```python
from build123d import *

# Parameters (mm, degrees)
F0_W        = 25
F0_H        = 25
F1_DEPTH    = 6
F2_W        = 13
F2_H        = 3
F3_DEPTH    = 25
F4_T1_DEPTH = 50.7168298797
F4_T3_DEPTH = 50.7168298797


# Not quite as in the source:
# - a fillet or chamfer that OpenCascade refuses, or shapes differently, is made with other operations: its cross-section is extruded or revolved along the edge and cut away or added


with BuildPart() as f1:
    # F0 (on Top) → F1 (new body)
    with BuildSketch(Plane.XY):
        with Locations((-12.5, 12.5)):
            Rectangle(F0_W, F0_H)
    extrude(amount=F1_DEPTH)

    # F2 (on face) → F3 (cut)
    with BuildSketch(Plane(origin=(-25, 0, 0), x_dir=(0, -1, 0), z_dir=(-1, 0, 0))):
        with Locations((-12.5, 3)):
            Rectangle(F2_W, F2_H)
    extrude(amount=-F3_DEPTH, mode=Mode.SUBTRACT)

    # F4: chamfer of 5 on 4 edges, made by hand

    # F4_s2 → F4_t1 (cut)
    with BuildSketch(Plane.YZ.offset(-37.8584149398)):
        Polygon((0, 1), (5, 6), (0, 6), align=None)
        Polygon((20, 6), (25, 1), (25, 6), align=None)
    extrude(amount=F4_T1_DEPTH, mode=Mode.SUBTRACT)

    # F4_s4 → F4_t3 (cut)
    with BuildSketch(Plane.XZ.offset(-37.8584149398)):
        Polygon((-25, 1), (-20, 6), (-25, 6), align=None)
        Polygon((0, 1), (-5, 6), (0, 6), align=None)
    extrude(amount=F4_T3_DEPTH, mode=Mode.SUBTRACT)


solid = f1.part
```
CAD build for the part. Positions are in the model's coordinates, mm. A direction names the side the tool comes from. Round coordinates to 2 decimals unless told otherwise and drop trailing zeros. Loops run counter-clockwise (first coordinate to the right, second up) from the corner with the lowest first, then second, coordinate; pieces in that order, holes last. Notation, with made-up numbers: M 76.5,64.25 L 100.5,64.25 A12 cw 100.5,77.25 Z; hole C 70,84 d7. An arc over 180 degrees is marked long. Return JSON: item names as keys, results as strings. Group by question number.
(1) Saw through at C-C, the plane x = -22.25. List the corners of the cut face in (y, z).
(2) Saw through at B-B, the plane z = 3.75. List the corners of the cut face in (x, y), and give its area (3 significant figures).
(3) Mould opens along Y. For faces 1 (the flat face through (-13, 13, 1.5)), 2 (the flat face through (-4, 13, 5)), 3 (the flat face through (-13, 22, 4)), 4 (the flat face through (-13, 2, 3)) say: +Y half, -Y half, draft (parallel to the pull), parting line (faces both ways), or undercut.
(4) Saw through at D-D, the plane x = -11.5. List the corners of the cut face in (y, z).
(5) Saw through at A-A, the plane y = 12.25. List the corners of the cut face in (x, z), and give its area (3 significant figures).
(6) Wall check: probe 1 along Z at (x, y) = (-15.5, 7.5); probe 2 along Z at (x, y) = (-22.75, 15); probe 3 along Z at (x, y) = (-18.75, 21.5). Give the ranges that are in metal, low to high. Write a range as [from, to].
(7) Tool access for faces 5 (the flat face through (-13, 19, 3)), 6 (the flat face through (-13, 13, 0)): list every direction of +Z, -Z, +X, -X, +Y, -Y with a clear straight run to the whole face (end or side of a thin tool).
(8) Drop flat-ended pins along their axis: P1, Ø2.5, axis at x = -6.5, z = 2.5, coming from the -Y side; P2, Ø1.5, axis at x = -22.5, z = 3, coming from the -Y side. Give the stop position or say it passes through.
Answer list:
{
 "1": {"outline": "M 0,0 L 25,0 L 25,1 L 22.25,3.75 L 19,3.75 L 19,1.5 L 6,1.5 L 6,3.75 L 2.75,3.75 L 0,1 Z"},
 "2": {"outline": "M -22.25,2.75 L -2.75,2.75 L -2.75,6 L -22.25,6 Z; M -22.25,19 L -2.75,19 L -2.75,22.25 L -22.25,22.25 Z", "area": "127 mm2"},
 "3": {"face 1": "undercut", "face 2": "draft", "face 3": "+Y half", "face 4": "-Y half"},
 "4": {"outline": "M 0,0 L 25,0 L 25,1 L 20,6 L 5,6 L 0,1 Z; hole M 6,1.5 L 19,1.5 L 19,4.5 L 6,4.5 Z"},
 "5": {"outline": "M -25,0 L 0,0 L 0,1 L -0.5,1.5 L -24.5,1.5 L -25,1 Z; M -21.5,4.5 L -3.5,4.5 L -5,6 L -20,6 Z", "area": "62.0 mm2"},
 "6": {"probe 1": "[0, 1.5], [4.5, 6]", "probe 2": "[0, 1.5]", "probe 3": "[0, 4.5]"},
 "7": {"face 5": "+X, -X", "face 6": "-Z, +X, -X, +Y, -Y"},
 "8": {"P1": "y = 0.25", "P2": "y = 1.25"}
}
